For this review, take the finished solid that the model builds, in its own axes (mm). A direction names the side the tool comes from. Round coordinates to 2 decimals unless told otherwise and drop trailing zeros. Order: outer loops, then holes, each group sorted by start corner. A loop starts at its lowest first (then second) coordinate and runs counter-clockwise, first axis right, second up. Notation, with made-up numbers: (78.25, 15.25) - (104.25, 15.25) arc R27 ccw to (104.25, 50.25) - close; hole circle Ø11 at (71, 58.5). An arc over 180 degrees is marked (long way). Write each question's results on one line, items separated by ' | '. Start each with the question number.
(1) For L1, parallel to Z at x = -16, y = -1.85; L2, parallel to Z at x = 16, y = 0.05, list the stretches that pass through material, from the lowest coordinate up. Write a range as from..to.
(2) For faces 1 (the cylindrical face through (18.48, -1.71, 19.14)), 2 (the cylindrical face through (0, 1, 20)), list the 3-axis set-ups (+Z, -Z, +X, -X, +Y, -Y) from which the entire face can be reached by the end or side of a thin tool; tool diameter is ignored.
(3) Take a section at B-B, the plane x = -16. Give the boundary of the cut face in (y, z), plus the area to 3 significant figures.
(4) Insertion check: pin 1 Ø2 at (x, y) = (-6, 0) entering from +Z; pin 2 Ø2 at (y, z) = (-2, -11.5) entering from -X; pin 3 Ø2 at (x, z) = (3, -14) entering from -Y. Each pin has a flat end and moves straight along its axis. Give the tip position at first contact, or say it passes through.
(5) Draft analysis for pull direction X (two halves, no side actions). For faces 3 (the cylindrical face through (-20, 1, 0)), 4 (the cylindrical face through (0, 1, -20)), 5 (the cylindrical face through (20, 1, 0)), 6 (the flat face through (-14, -4, -16)), state which applies: pulls with the +X half, pulls with the -X half, needs draft (parallel to the pull), parting line crosses it, or undercut.
(6) Take a section at A-A, the plane y = -1. Give the boundary of the cut face in (x, z).
(7) Take a section at C-C, the plane z = 16. Give the boundary of the cut face in (x, y), plus the area to 3 significant figures.
(8) Take a section at D-D, the plane x = 13.5. Give the boundary of the cut face in (y, z).
```python
from build123d import *

# Parameters (mm, degrees)
SKETCH1_R                  = 4
SKETCH1_R_2                = 20
BOSS_EXTRUDE1_DEPTH        = 2
FILLET1_R                  = 3
BOSS_EXTRUDE2_START        = -4
SKETCH1_3_R                = 4
BOSS_EXTRUDE2_DEPTH        = 4
F_3_5_3_5_DIAMETER_HOLE1_D = 3.5


with BuildPart() as part:
    # Sketch1 → Boss-Extrude1 (new body)
    with BuildSketch(Plane(origin=(0, 0, 0), x_dir=(1, 0, 0), z_dir=(0, 1, 0))):
        with Locations((-16, -16)):
            Circle(SKETCH1_R)
        Circle(SKETCH1_R_2)
        with Locations((16, -16)):
            Circle(SKETCH1_R)
        with Locations((16, 16)):
            Circle(SKETCH1_R)
        with Locations((-16, 16)):
            Circle(SKETCH1_R)
    extrude(amount=BOSS_EXTRUDE1_DEPTH)

    # Fillet1
    fillet1_edges = [part.edges().sort_by_distance(p)[0] for p in [
        (-16, 1, 12),
        (-16, 1, -12),
        (-12, 1, -16),
        (12, 1, -16),
        (16, 1, -12),
        (16, 1, 12),
        (12, 1, 16),
        (-12, 1, 16),
    ]]
    fillet(fillet1_edges, radius=FILLET1_R)

    # Sketch1_3 → Boss-Extrude2 (add)
    with BuildSketch(Plane(origin=(0, 0, 0), x_dir=(1, 0, 0), z_dir=(0, 1, 0)).offset(BOSS_EXTRUDE2_START)):
        with Locations(Location((-16, 16, 0), (0, 0, 39.20236367))):
            Circle(SKETCH1_3_R)
        with Locations(Location((16, 16, 0), (0, 0, 140.79763633))):
            Circle(SKETCH1_3_R)
        with Locations(Location((16, -16, 0), (0, 0, 50.79763633))):
            Circle(SKETCH1_3_R)
        with Locations(Location((-16, -16, 0), (0, 0, 129.20236367))):
            Circle(SKETCH1_3_R)
    extrude(amount=BOSS_EXTRUDE2_DEPTH)

    # 3.5 _3.5_ Diameter Hole1 (through all)
    with Locations(Plane(origin=(0, 2, 0), x_dir=(1, 0, 0), z_dir=(0, 1, 0))):
        with Locations((-16, 16), (16, 16), (16, -16), (-16, -16)):
            Hole(F_3_5_3_5_DIAMETER_HOLE1_D / 2)


solid = part.part
```
Results below:
1) L1: z = -20..-17.75, -14.25..-12, 12..14.25, 17.75..20 | L2: z = -20..-17.75, -14.25..14.25, 17.75..20
2) face 1: -Y | face 2: +Z, +Y, -Y
3) outline: (-4, -20) - (2, -20) - (2, -17.75) - (-4, -17.75) - close; (-4, -14.25) - (2, -14.25) - (2, 14.25) - (-4, 14.25) - (-4, 12) - (0, 12) - (0, -12) - (-4, -12) - close; (-4, 17.75) - (2, 17.75) - (2, 20) - (-4, 20) - close | area: 102 mm^2
4) pin 1: stops at z = 19.36 | pin 2: stops at x = -17.94 | pin 3: stops at y = 0
5) face 3: pulls with the -X half | face 4: undercut | face 5: pulls with the +X half | face 6: needs draft
6) outline: circle Ø8 at (-16, -16); circle Ø8 at (-16, 16); circle Ø8 at (16, -16); circle Ø8 at (16, 16); hole circle Ø3.5 at (-16, -16); hole circle Ø3.5 at (-16, 16); hole circle Ø3.5 at (16, -16); hole circle Ø3.5 at (16, 16)
7) outline: (-20, -4) - (-17.75, -4) - (-17.75, 2) - (-20, 2) - close; (-14.25, -4) - (-12, -4) - (-12, 0) - (12, 0) - (12, -4) - (14.25, -4) - (14.25, 2) - (-14.25, 2) - close; (17.75, -4) - (20, -4) - (20, 2) - (17.75, 2) - close | area: 102 mm^2
8) outline: (-4, -19.12) - (2, -19.12) - (2, 19.12) - (-4, 19.12) - (-4, 12.88) - (0, 12.88) - (0, -12.88) - (-4, -12.88) - close
